Part model, mm, in its own coordinate system. Give positions to 0.01 mm unless a question says otherwise; leave off trailing zeros. Order: outer loops, then holes, each group sorted by start corner. A loop starts at its lowest first (then second) coordinate and runs counter-clockwise, first axis right, second up. Notation, with made-up numbers: M 75.5,5.5 L 91.5,5.5 A36 ccw 91.5,41.5 Z; hole C -28,43 d4. An arc over 180 degrees is marked long. Answer as a JSON object with one key per item and string values.
from build123d import *

# Parameters (mm, degrees)
SKETCH_1_R      = 13.5
SKETCH_1_R_2    = 1.6
SKETCH_1_R_3    = 2.15
EXTRUDE_1_DEPTH = 5


with BuildPart() as part:
    # ｽｹｯﾁ1 → ﾎﾞｽ - 押し出し1 (new body)
    with BuildSketch(Plane(origin=(0, 0, 0), x_dir=(1, 0, 0), z_dir=(0, 1, 0))):
        with BuildLine():
            ThreePointArc((15.151339784, 22.006829374), (11.924552334, 19.398069264), (7.776551803, 19.507056212))
            ThreePointArc((7.776551803, 19.507056212), (-14.849242405, 14.849242405), (-19.507056212, -7.776551803))
            ThreePointArc((-19.507056212, -7.776551803), (-19.398069264, -11.924552334), (-22.006829374, -15.151339784))
            ThreePointArc((-22.006829374, -15.151339784), (-22.980970389, -22.980970389), (-15.151339784, -22.006829374))
            ThreePointArc((-15.151339784, -22.006829374), (-11.924552334, -19.398069264), (-7.776551803, -19.507056212))
            ThreePointArc((-7.776551803, -19.507056212), (0, -21), (7.776551803, -19.507056212))
            ThreePointArc((7.776551803, -19.507056212), (11.924552334, -19.398069264), (15.151339784, -22.006829374))
            ThreePointArc((15.151339784, -22.006829374), (22.980970389, -22.980970389), (22.006829374, -15.151339784))
            ThreePointArc((22.006829374, -15.151339784), (19.398069264, -11.924552334), (19.507056212, -7.776551803))
            ThreePointArc((19.507056212, -7.776551803), (21, 0), (19.507056212, 7.776551803))
            ThreePointArc((19.507056212, 7.776551803), (19.398069264, 11.924552334), (22.006829374, 15.151339784))
            ThreePointArc((22.006829374, 15.151339784), (22.980970389, 22.980970389), (15.151339784, 22.006829374))
        make_face()
        with Locations(Location((0, 0, 0), (0, 0, 270))):
            Circle(SKETCH_1_R, mode=Mode.SUBTRACT)
        with Locations(Location((12.374368671, 12.374368671, 0), (0, 0, 270))):
            Circle(SKETCH_1_R_2, mode=Mode.SUBTRACT)
        with Locations(Location((12.374368671, -12.374368671, 0), (0, 0, 270))):
            Circle(SKETCH_1_R_2, mode=Mode.SUBTRACT)
        with Locations(Location((-12.374368671, -12.374368671, 0), (0, 0, 270))):
            Circle(SKETCH_1_R_2, mode=Mode.SUBTRACT)
        with Locations(Location((-12.374368671, 12.374368671, 0), (0, 0, 270))):
            Circle(SKETCH_1_R_2, mode=Mode.SUBTRACT)
        with Locations(Location((19.445436483, 19.445436483, 0), (0, 0, 270))):
            Circle(SKETCH_1_R_3, mode=Mode.SUBTRACT)
        with Locations(Location((19.445436483, -19.445436483, 0), (0, 0, 270))):
            Circle(SKETCH_1_R_3, mode=Mode.SUBTRACT)
        with Locations(Location((-19.445436483, -19.445436483, 0), (0, 0, 270))):
            Circle(SKETCH_1_R_3, mode=Mode.SUBTRACT)
    extrude(amount=EXTRUDE_1_DEPTH)


solid = part.part
1. Cut at A-A on x = 0. Give the cut face in (y, z).
Worked answers:
{"outline": "M 0,-21 L 5,-21 L 5,-13.5 L 0,-13.5 Z; M 0,13.5 L 5,13.5 L 5,21 L 0,21 Z"}
2. Cut at B-B on z = 0. Give the cut face in (x, y).
Worked answers:
{"outline": "M -21,0 L -13.5,0 L -13.5,5 L -21,5 Z; M 13.5,0 L 21,0 L 21,5 L 13.5,5 Z"}
3. Pin check, flat tips, straight feed: P1, Ø3, axis at y = 4, z = 9, coming from the +X side; P2, Ø2, axis at x = -7, y = 0.5, coming from the -Z side. Stop position of each tip, or through.
Worked answers:
{"P1": "stops at x = 19.62", "P2": "stops at z = -20.12"}
4. Two-plate mould, pull along Z, no slides. Class faces 1 (the cylindrical face through (-11.981, 2.465, 19.417)), 2 (the flat face through (11, 5, 11)), 3 (the cylindrical face through (-17.314, 2.465, 19.166)), 4 (the cylindrical face through (21, 2, 0)): +Z half, -Z half, draft (parallel to the pull), parting line (faces both ways), or undercut.
Worked answers:
{"face 1": "+Z half", "face 2": "draft", "face 3": "undercut", "face 4": "undercut"}
5. Probe line 1 along X through (y, z) = (1.5, -0.5); line 2 along Z through (x, y) = (-19, 4.3); line 3 along Z through (x, y) = (-3, 4.2). List the from-to ranges inside material, lowest first.
Worked answers:
{"line 1": "x = -20.99 to -13.49, 13.49 to 20.99", "line 2": "z = -8.94 to 17.34, 21.55 to 24.43", "line 3": "z = -20.78 to -13.16, 13.16 to 20.78"}
6. Cut at C-C on y = 2.45. State how many separate pieces and enclosed holes the cut face has, plus the area to 3 significant figures.
Worked answers:
{"separate pieces": "1", "enclosed holes": "8", "area": "1,060 mm^2"}
